from build123d import *

# Parameters (mm, degrees)
F1_DEPTH  = 50.8
F3_DEPTH  = 6.35
F3_FACE_W = 6.35
F3_FACE_H = 6.35
F4_DEPTH  = 25.4
F5_W      = 6.35
F5_H      = 6.35
F6_DEPTH  = 25.4


with BuildPart() as f1:
    # F0 (on Front) → F1 (new body)
    with BuildSketch(Plane.XZ):
        Polygon((-12.7, 0), (-6.35, 0), (-9.525, 3.175), (-9.525, 6.35), (0, 6.35), (9.525, 6.35), (9.525, 3.175), (6.35, 0), (12.7, 0), (12.7, 12.7), (0, 12.7), (-12.7, 12.7), align=None)
    extrude(amount=-F1_DEPTH)

    # F2 (on face) → F3 (join)
    with BuildSketch(Plane(origin=(-12.7, 0, 0), x_dir=(0, -1, 0), z_dir=(-1, 0, 0))):
        Polygon((-22.225, 9.525), (-25.4, 9.525), (-28.575, 9.525), (-28.575, 3.175), (-22.225, 3.175), align=None)
    extrude(amount=F3_DEPTH)

    # F3_face (on face) → F4 (join)
    with BuildSketch(Plane(origin=(-15.875, 25.4, 3.175), x_dir=(1, 0, 0), z_dir=(0, 0, -1))):
        Rectangle(F3_FACE_W, F3_FACE_H)
    extrude(amount=F4_DEPTH)

    # F5 (on face) → F6 (join)
    with BuildSketch(Plane.XZ.offset(-22.225)):
        with Locations((-15.875, -19.05)):
            Rectangle(F5_W, F5_H)
    extrude(amount=F6_DEPTH)


solid = f1.part
CAD build for the part. Positions are in the model's coordinates, mm. A direction names the side the tool comes from. Coordinates: 2 decimals unless noted, no trailing zeros. Order: outer loops, then holes, each group sorted by start corner. A loop starts at its lowest first (then second) coordinate and runs counter-clockwise, first axis right, second up.
Item 1: Two-plate mould, pull along Z, no slides. Class faces 4 (the face through (9.525, 25, 5)), 5 (the face through (9, 25, 0)), 6 (the face through (0, 25, 12.7)): +Z half, -Z half, draft (parallel to the pull), parting line (faces both ways), or undercut.
Check sheet entries:
face 4: undercut
face 5: -Z half
face 6: +Z half
Item 2: Drill centre lines: L1, parallel to X at y = 5, z = 4.5 (3 decimals); L2, parallel to Z at x = -4, y = 11.5; L3, parallel to X at y = 23.5, z = -10. Where is each one in solid material? Low to high.
Check sheet entries:
L1: x = -12.7 to -9.525, 9.525 to 12.7
L2: z = 6.35 to 12.7
L3: x = -19.05 to -12.7
Item 3: Band-saw the part on A-A on y = 9. List the corners of the cut face in (x, z) (3 decimals), plus the area to 3 significant figures.
Check sheet entries:
outline: (-19.05, -22.225) - (-12.7, -22.225) - (-12.7, -15.875) - (-19.05, -15.875) - close; (-12.7, 0) - (-6.35, 0) - (-9.525, 3.175) - (-9.525, 6.35) - (9.525, 6.35) - (9.525, 3.175) - (6.35, 0) - (12.7, 0) - (12.7, 12.7) - (-12.7, 12.7) - close
area: 252 mm2
Item 4: 3-axis set-ups, long thin cutter, end or side, ignore diameter. For faces 1 (the face through (-12.7, 16.5, -16.2)), 2 (the face through (-16, 25, 9.525)), 3 (the face through (-9.525, 25, 5)): which of +Z, -Z, +X, -X, +Y, -Y reach the whole face in a straight line?
Check sheet entries:
face 1: -Z, +X, +Y, -Y
face 2: +Z, -X, +Y, -Y
face 3: +Y, -Y
Item 5: Band-saw the part on B-B on z = 1. List the corners of the cut face in (x, y) (3 decimals).
Check sheet entries:
outline: (-19.05, 22.225) - (-12.7, 22.225) - (-12.7, 0) - (-7.35, 0) - (-7.35, 50.8) - (-12.7, 50.8) - (-12.7, 28.575) - (-19.05, 28.575) - close; (7.35, 0) - (12.7, 0) - (12.7, 50.8) - (7.35, 50.8) - close
Item 6: Band-saw the part on C-C on x = 8.5. List the corners of the cut face in (y, z), plus the area to 3 significant figures.
Check sheet entries:
outline: (0, 0) - (50.8, 0) - (50.8, 2.15) - (0, 2.15) - close; (0, 6.35) - (50.8, 6.35) - (50.8, 12.7) - (0, 12.7) - close
area: 432 mm2
Item 7: Pin check, flat tips, straight feed: pin 1 Ø1.5 at (x, y) = (-9, 29) entering from -Z; pin 2 Ø3 at (x, z) = (-16.5, -9.5) entering from -Y (3 decimals); pin 3 Ø5 at (x, y) = (-16, 5) entering from +Z (3 decimals). Stop position of each tip, or through.
Check sheet entries:
pin 1: stops at z = 0
pin 2: stops at y = 22.225
pin 3: stops at z = -15.875
Item 8: Band-saw the part on D-D on y = 44. List the corners of the cut face in (x, z) (3 decimals), plus the area to 3 significant figures.
Check sheet entries:
outline: (-12.7, 0) - (-6.35, 0) - (-9.525, 3.175) - (-9.525, 6.35) - (9.525, 6.35) - (9.525, 3.175) - (6.35, 0) - (12.7, 0) - (12.7, 12.7) - (-12.7, 12.7) - close
area: 212 mm2
